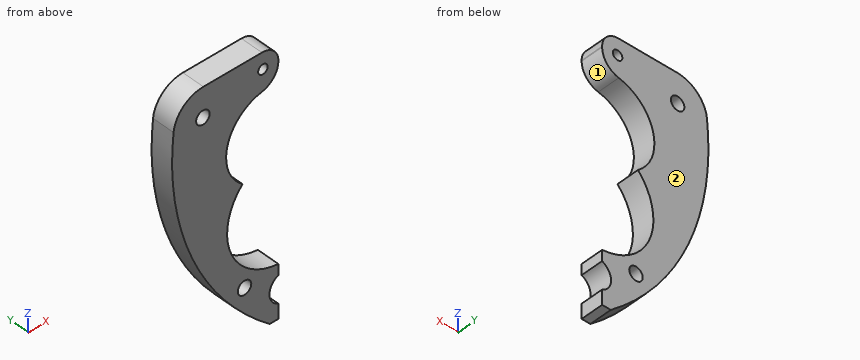
```python
from build123d import *

# Parameters (mm, degrees)
BOSS_EXTRUDE1_DEPTH = 5.842
CUT_EXTRUDE1_DEPTH  = 77.930082101
CUT_EXTRUDE2_DEPTH  = 77.930082101
SKETCH8_R           = 11.43
CUT_EXTRUDE3_DEPTH  = 77.930082101
FILLET1_R           = 7.874
FILLET2_R           = 4.318
FILLET4_R           = 5.334
SKETCH9_R           = 1.774805699
CUT_EXTRUDE4_DEPTH  = 77.930082101
SKETCH10_R          = 1.25
CUT_EXTRUDE5_DEPTH  = 77.930082101
SKETCH11_R          = 1.778
CUT_EXTRUDE6_DEPTH  = 77.930082101


with BuildPart() as part:
    # Sketch1 → Boss-Extrude1 (new body)
    with BuildSketch(Plane(origin=(0, 0, 0), x_dir=(1, 0, 0), z_dir=(0, 1, 0))):
        with BuildLine():
            Line((30.379802604, 69.40499916), (32.665802604, 69.40499916))
            Line((32.665802604, 69.40499916), (32.665802604, 0.57099916))
            Line((32.665802604, 0.57099916), (6.249802604, 0.57099916))
            ThreePointArc((6.249802604, 0.57099916), (8.73869024, 38.344938918), (30.379802604, 69.40499916))
        make_face()
    extrude(amount=BOSS_EXTRUDE1_DEPTH)

    # Sketch2 → Cut-Extrude1 (cut, through all)
    with BuildSketch(Plane(origin=(0, 5.842, 0), x_dir=(1, 0, 0), z_dir=(0, 1, 0))):
        with BuildLine():
            Line((32.665802604, 65.59499916), (32.665802604, 58.48299916))
            ThreePointArc((32.665802604, 58.48299916), (30.320989866, 62.03899916), (32.665802604, 65.59499916))
        make_face()
    extrude(amount=-CUT_EXTRUDE1_DEPTH, mode=Mode.SUBTRACT)

    # Sketch7 → Cut-Extrude2 (cut, through all)
    with BuildSketch(Plane(origin=(0, 5.842, 0), x_dir=(1, 0, 0), z_dir=(0, 1, 0))):
        with BuildLine():
            Line((32.665802604, 55.68899916), (32.665802604, 25.872384999))
            ThreePointArc((32.665802604, 25.872384999), (19.203802604, 40.780692079), (32.665802604, 55.68899916))
        make_face()
    extrude(amount=-CUT_EXTRUDE2_DEPTH, mode=Mode.SUBTRACT)

    # Sketch8 → Cut-Extrude3 (cut, through all)
    with BuildSketch(Plane(origin=(0, 5.842, 0), x_dir=(1, 0, 0), z_dir=(0, 1, 0))):
        with Locations((30.379802604, 21.612613445)):
            Circle(SKETCH8_R)
    extrude(amount=-CUT_EXTRUDE3_DEPTH, mode=Mode.SUBTRACT)

    # Fillet1
    fillet1_edges = [part.edges().sort_by_distance(p)[0] for p in [
        (6.249802604, 2.921, -0.57099916),
    ]]
    fillet(fillet1_edges, radius=FILLET1_R)

    # Fillet2
    fillet2_edges = [part.edges().sort_by_distance(p)[0] for p in [
        (32.665802604, 2.921, -0.57099916),
    ]]
    fillet(fillet2_edges, radius=FILLET2_R)

    # Fillet4
    fillet4_edges = [part.edges().sort_by_distance(p)[0] for p in [
        (32.665802604, 2.921, -10.413546341),
    ]]
    fillet(fillet4_edges, radius=FILLET4_R)

    # Sketch9 → Cut-Extrude4 (cut, through all)
    with BuildSketch(Plane(origin=(0, 5.842, 0), x_dir=(1, 0, 0), z_dir=(0, 1, 0))):
        with Locations(Location((23.775802604, 56.70499916, 0), (0, 0, 270))):
            Circle(SKETCH9_R)
    extrude(amount=-CUT_EXTRUDE4_DEPTH, mode=Mode.SUBTRACT)

    # Sketch10 → Cut-Extrude5 (cut, through all)
    with BuildSketch(Plane(origin=(0, 5.842, 0), x_dir=(1, 0, 0), z_dir=(0, 1, 0))):
        with Locations(Location((28.601802604, 4.88899916, 0), (0, 0, 270))):
            Circle(SKETCH10_R)
    extrude(amount=-CUT_EXTRUDE5_DEPTH, mode=Mode.SUBTRACT)

    # Sketch11 → Cut-Extrude6 (cut, through all)
    with BuildSketch(Plane(origin=(0, 5.842, 0), x_dir=(1, 0, 0), z_dir=(0, 1, 0))):
        with Locations(Location((12.853802604, 8.19099916, 0), (0, 0, 270))):
            Circle(SKETCH11_R)
    extrude(amount=-CUT_EXTRUDE6_DEPTH, mode=Mode.SUBTRACT)


solid = part.part
```
Build history of the part. All positions in model axes, mm. Face numbers are marked on the shaded views. A direction names the side the tool comes from. Coordinates: 2 decimals unless noted, no trailing zeros. Write each loop counter-clockwise with the first axis right and the second up, starting at its lowest first coordinate (ties: lowest second). Pieces come first, ordered by that corner, then holes.
1. Band-saw the part on A-A, the plane x = 24.5. Give the cut face in (y, z), and give its area (3 significant figures).
Answer block:
outline: (0, -63.95) - (5.84, -63.95) - (5.84, -58.33) - (0, -58.33) - close; (0, -55.08) - (5.84, -55.08) - (5.84, -52.21) - (0, -52.21) - close; (0, -11.81) - (5.84, -11.81) - (5.84, -0.57) - (0, -0.57) - close
area: 115 mm2
2. Band-saw the part on B-B, the plane y = 2.85. Give the cut face in (x, z) (3 decimals), and give its area (3 significant figures).
Answer block:
outline: (5.148, -7.624) arc R70.612 ccw to (30.38, -69.405) - (32.666, -69.405) - (32.666, -65.595) arc R3.869 cw to (32.666, -58.483) - (32.666, -55.689) arc R14.986 cw to (23.246, -30.543) arc R11.43 cw to (28.302, -10.373) arc R5.334 ccw to (32.666, -5.128) - (32.666, -4.889) arc R4.318 ccw to (28.348, -0.571) - (12.979, -0.571) arc R7.874 ccw to start; hole circle Ø3.556 at (12.854, -8.191); hole circle Ø3.55 at (23.776, -56.705); hole circle Ø2.5 at (28.602, -4.889)
area: 916 mm2
3. Band-saw the part on C-C, the plane x = 20.5. Give the cut face in (y, z), and give its area (3 significant figures).
Answer block:
outline: (0, -59.42) - (5.84, -59.42) - (5.84, -46.88) - (0, -46.88) - close; (0, -34.68) - (5.84, -34.68) - (5.84, -27.36) - (0, -27.36) - close; (0, -15.87) - (5.84, -15.87) - (5.84, -0.57) - (0, -0.57) - close
area: 205 mm2
4. Drill centre lines: probe 1 along Z at (x, y) = (23.5, 5.3) (3 decimals); probe 2 along Z at (x, y) = (23, 5.3); probe 3 along Z at (x, y) = (31, 2.1) (3 decimals). Where is each one in solid material? Low to high.
Answer block:
probe 1: z = -62.892 to -58.458, -54.952 to -51.283, -12.485 to -0.571
probe 2: z = -62.34 to -58.3, -55.11 to -50.75, -30.81 to -30.34, -12.88 to -0.57
probe 3: z = -69.405 to -64.228, -59.85 to -55.423, -9 to -1.482
5. Drop flat-ended pins along their axis: pin 1 (3 mm diameter, centred on x = 23.78, z = -56.7, fed in from +Y); pin 2 (3 mm diameter, centred on y = 3.5, z = -38.5, fed in from +X). Give the stop position or say it passes through.
Answer block:
pin 1: passes through
pin 2: stops at x = 19.69
6. Band-saw the part on D-D, the plane z = -42.5. Give the cut face in (x, y), and give its area (3 significant figures).
Answer block:
outline: (10.34, 0) - (19.3, 0) - (19.3, 5.84) - (10.34, 5.84) - close
area: 52.3 mm2
7. 3-axis set-ups, long thin cutter, end or side, ignore diameter. For the marked faces 1 and 2: which of +Z, -Z, +X, -X, +Y, -Y reach the whole face in a straight line?
Answer block:
face 1: +X, +Y, -Y
face 2: +Z, -Z, +X, -X, +Y
